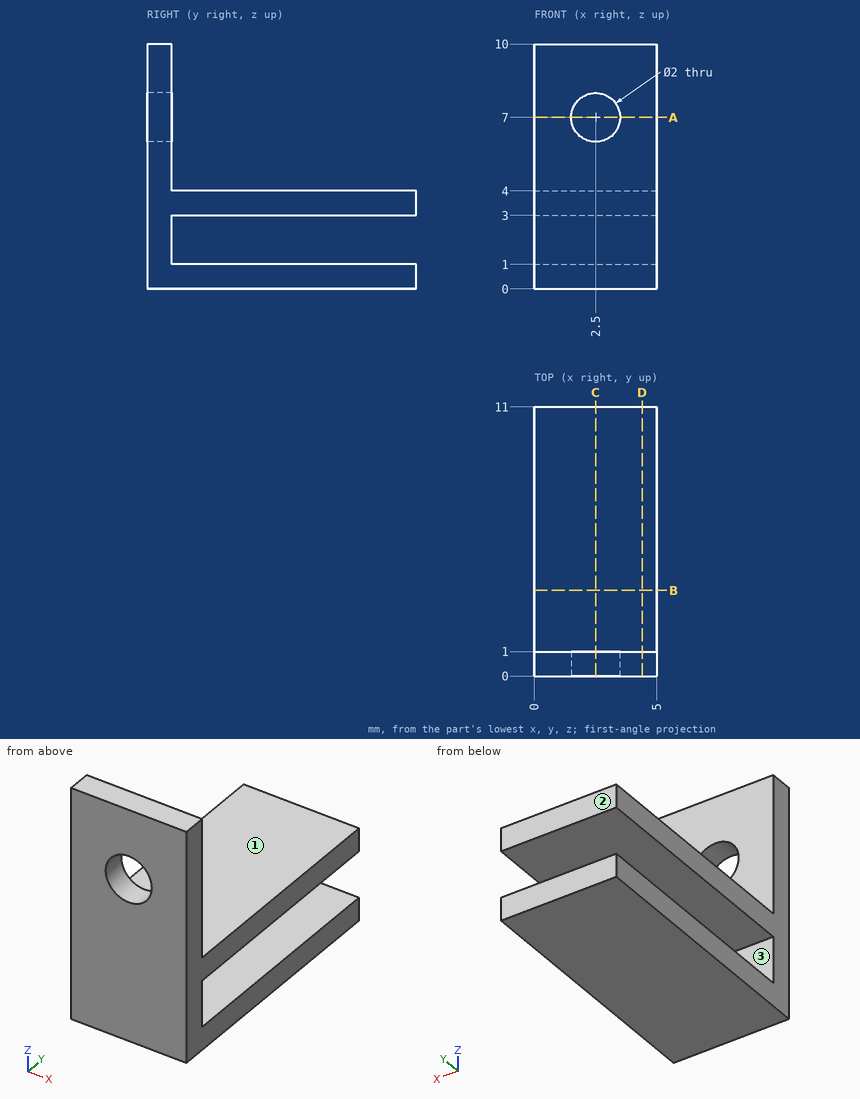
Print and shaded views of the part. All mm, measured from the part's lowest x, y and z. A direction names the side the tool comes from. Round coordinates to 2 decimals unless told otherwise and drop trailing zeros. Write each loop counter-clockwise with the first axis right and the second up, starting at its lowest first coordinate (ties: lowest second). Pieces come first, ordered by that corner, then holes. Notation, with made-up numbers: M -10.75,2.25 L 11.25,2.25 A16 ccw 11.25,16.25 Z; hole C 25.5,12.5 d10. An arc over 180 degrees is marked long. Use a Markdown table: item, result. Add a question column.
1. Slice it at D-D on x = 4.4. Give the cut face in (y, z), then the cut area to 3 significant figures.
2. 3-axis set-ups, long thin cutter, end or side, ignore diameter. For the marked faces 1, 2 and 3: which of +Z, -Z, +X, -X, +Y, -Y reach the whole face in a straight line?
3. Drill centre lines: probe 1 along X at (y, z) = (0.25, 7); probe 2 along Z at (x, y) = (2.5, 0.5); probe 3 along Z at (x, y) = (4.2, 9). Where is each one in solid material? Low to high.
4. Slice it at A-A on z = 7. Give the cut face in (x, y), then the cut area to 3 significant figures.
5. Flat gauge pins, fed straight in: P1, Ø2.5, axis at x = 3, y = 3.5, coming from the +Z side; P2, Ø1.2, axis at x = 2.5, z = 7, coming from the -Y side. Where does each tip first touch, or does it go through?
6. Slice it at B-B on y = 3.5. Give the cut face in (x, z).
7. Slice it at C-C on x = 2.5. Give the cut face in (y, z), then the cut area to 3 significant figures.
Reply:
| question | item | result |
|---|---|---|
| 1 | outline | M 0,0 L 11,0 L 11,1 L 1,1 L 1,3 L 11,3 L 11,4 L 1,4 L 1,10 L 0,10 Z |
| 1 | area | 30.0 mm^2 |
| 2 | face 1 | +Z, +X, -X, +Y |
| 2 | face 2 | +Z, -Z, +X, -X, +Y |
| 2 | face 3 | +X, -X, +Y |
| 3 | probe 1 | x = 0 to 1.5, 3.5 to 5 |
| 3 | probe 2 | z = 0 to 6, 8 to 10 |
| 3 | probe 3 | z = 0 to 1, 3 to 4 |
| 4 | outline | M 0,0 L 1.5,0 L 1.5,1 L 0,1 Z; M 3.5,0 L 5,0 L 5,1 L 3.5,1 Z |
| 4 | area | 3.00 mm^2 |
| 5 | P1 | stops at z = 4 |
| 5 | P2 | passes through |
| 6 | outline | M 0,0 L 5,0 L 5,1 L 0,1 Z; M 0,3 L 5,3 L 5,4 L 0,4 Z |
| 7 | outline | M 0,0 L 11,0 L 11,1 L 1,1 L 1,3 L 11,3 L 11,4 L 1,4 L 1,6 L 0,6 Z; M 0,8 L 1,8 L 1,10 L 0,10 Z |
| 7 | area | 28.0 mm^2 |
